Job drawing, mm, ordinate dimensions from the low corner. One solid piece. A direction names the side the tool comes from. Coordinates: 2 decimals unless noted, no trailing zeros. Write each loop counter-clockwise with the first axis right and the second up, starting at its lowest first coordinate (ties: lowest second). Pieces come first, ordered by that corner, then holes.
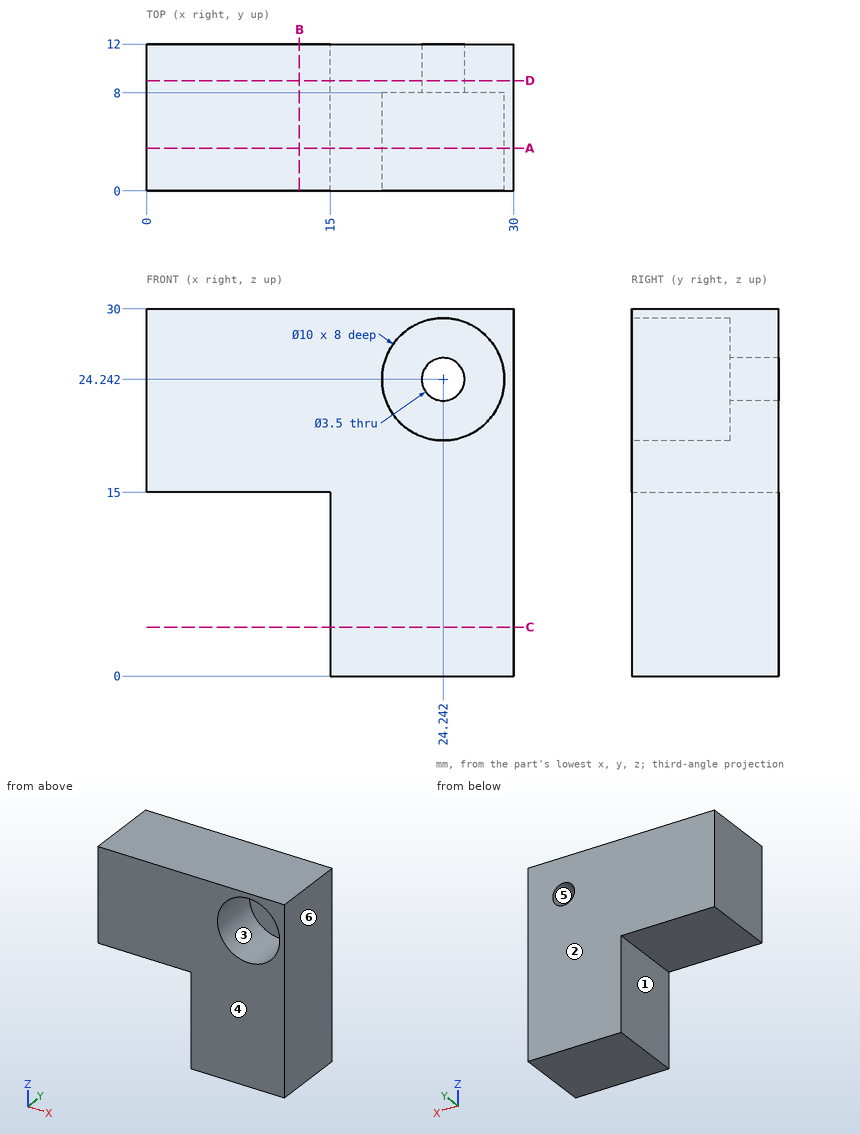
1. Mould opens along X. For the marked faces 4, 5 and 6 say: +X half, -X half, draft (parallel to the pull), parting line (faces both ways), or undercut.
Computed values:
face 4: draft
face 5: undercut
face 6: +X half
2. Saw through at B-B on x = 12.5. List the corners of the cut face in (y, z), plus the area to 3 significant figures.
Computed values:
outline: (0, 15) - (12, 15) - (12, 30) - (0, 30) - close
area: 180 mm2
3. 3-axis set-ups, long thin cutter, end or side, ignore diameter. For the marked faces 1, 2 and 3: which of +Z, -Z, +X, -X, +Y, -Y reach the whole face in a straight line?
Computed values:
face 1: -Z, -X, +Y, -Y
face 2: +Z, -Z, +X, -X, +Y
face 3: -Y
4. Saw through at C-C on z = 4. List the corners of the cut face in (x, y), plus the area to 3 significant figures.
Computed values:
outline: (15, 0) - (30, 0) - (30, 12) - (15, 12) - close
area: 180 mm2
5. Flat gauge pins, fed straight in: pin 1 (3 mm diameter, centred on x = 11.5, y = 5, fed in from -Z); pin 2 (6 mm diameter, centred on y = 10, z = 6.5, fed in from -X); pin 3 (3 mm diameter, centred on x = 24.5, z = 25.5, fed in from -Y). Where does each tip first touch, or does it go through?
Computed values:
pin 1: stops at z = 15
pin 2: stops at x = 15
pin 3: stops at y = 8
6. Saw through at A-A on y = 3.5. List the corners of the cut face in (x, z), plus the area to 3 significant figures.
Computed values:
outline: (0, 15) - (15, 15) - (15, 0) - (30, 0) - (30, 30) - (0, 30) - close; hole circle Ø10 at (24.24, 24.24)
area: 596 mm2
7. Saw through at D-D on y = 9. List the corners of the cut face in (x, z).
Computed values:
outline: (0, 15) - (15, 15) - (15, 0) - (30, 0) - (30, 30) - (0, 30) - close; hole circle Ø3.5 at (24.24, 24.24)
8. Probe line 1 along X through (y, z) = (6.5, 6); line 2 along Z through (x, y) = (27.25, 5.5); line 3 along Z through (x, y) = (21.5, 1.25). List the from-to ranges inside material, lowest first.
Computed values:
line 1: x = 15 to 30
line 2: z = 0 to 20.25, 28.24 to 30
line 3: z = 0 to 20.06, 28.42 to 30
